Read the model definition and answer for the solid it produces. Units are mm, in the model's axes. A direction names the side the tool comes from. Give positions to 0.01 mm unless a question says otherwise; leave off trailing zeros. Write each loop counter-clockwise with the first axis right and the second up, starting at its lowest first coordinate (ties: lowest second). Pieces come first, ordered by that corner, then holes. Notation, with made-up numbers: (-14.75, -38) -> (-10.75, -38) arc R25 cw to (-10.75, -4) -> close; hole circle Ø8 at (45, -11.75). An arc over 180 degrees is marked (long way). Answer as CSV lines item,"result". Start each with the question number.
1. For a pull along Z with two mould halves and no side action, classify faces 1 (the flat face through (-32.4, 9, -5.3)), 2 (the cylindrical face through (-3.09, 169.89, -4.61)), 3 (the cylindrical face through (-9.634, 5.916, -3.034)) as pulls with the +Z half, pulls with the -Z half, needs draft (parallel to the pull), parting line crosses it, or undercut.
2. The part is cut by section A-A, the plane x = -30.4. Determine the outline of the cut face in (y, z).
3. The part is cut by section D-D, the plane x = 32. Determine the outline of the cut face in (y, z), and give its area (3 significant figures).
4. Find the intervals of material crossed by line 1 (X direction, y = 10.1, z = 0); line 2 (X direction, y = 7, z = 0); line 3 (Z direction, x = -30, y = 10), in increasing order.
5. A tool of negligible diameter and unlimited length cuts with its end or side. For faces 4 (the cylindrical face through (-10.99, 12.27, 0.48)), 5 (the cylindrical face through (-9.634, 100.261, -3.034)), 6 (the flat face through (0, 13, 10.4)), from which of +Z, -Z, +X, -X, +Y, -Y can it reach the whole face along a straight path? Write none if from no direction.
6. Given pin 1 (8 mm diameter, centred on y = 142.5, z = -8, fed in from +X); pin 2 (1.5 mm diameter, centred on x = 8.5, z = -5, fed in from +Y) (3 decimals); pin 3 (3 mm diameter, centred on x = 0, y = 170, fed in from +Z), each flat-ended and moving along its own axis, determine where each tip first touches the part or whether it passes through.
7. The part is cut by section B-B, the plane y = 180. Determine the outline of the cut face in (x, z).
8. The part is cut by section C-C, the plane y = 145. Determine the outline of the cut face in (x, z).
Autodesk Inventor part; units mm, degrees
ref_plane "Płaszczyzna konstrukcyjna1" through (0, 13, 0) normal (0, -1, 0) x (1, 0, 0)
ref_plane "Płaszczyzna konstrukcyjna2" through (0, 12, 0) normal (0, -1, 0) x (1, 0, 0)
ref_plane "YZ Plane" through (0, 0, 0) normal (1, 0, 0) x (0, 1, 0)
sketch "Szkic1" plane through (0, 0, 0) normal (0, 1, 0) x (-1, 0, 0)
  circle A0 centre (0, 0) radius 10.1
  dimension "d0" = 20.2
extrude "Wyciągnięcie proste1" add sketch "Szkic1" along normal blind 200
ref_plane "Płaszczyzna konstrukcyjna1" through (0, 13, 0) normal (0, -1, 0) x (1, 0, 0)
sketch "Szkic2" plane through (0, 13, 0) normal (0, -1, 0) x (1, 0, 0)
  line L0 (0, 0) -> (30.4, 0)
  line L1 (0, 0) -> (30.4, 0) construction
  circle A0 centre (30.4, 0) radius 5.5
  line L2 (35.9, 0) -> (36.9, 0)
  line L3 (36.9, 0) -> (0, 0)
  line L4 (0, 0) -> (0, -6)
  line L5 (0, -6) -> (36.9, -6)
  line L6 (36.9, -6) -> (36.9, 0)
  line L7 (0, 0) -> (0, -16.4984)
  line L8 (0, 6) -> (36.9, 6)
  line L9 (36.9, 6) -> (36.9, 0)
  line L10 (0, 0) -> (-30.4, 0)
  line L11 (0, 0) -> (-30.4, 0) construction
  circle A1 centre (-30.4, 0) radius 5.5
  line L12 (-35.9, 0) -> (-36.9, 0)
  line L13 (-36.9, 0) -> (0, 0)
  line L14 (0, -6) -> (-36.9, -6)
  line L15 (0, 6) -> (-36.9, 6)
  line L16 (-36.9, 6) -> (-36.9, -6)
  line L17 (-24.9, 0) -> (-23.9, 0)
  line L18 (-23.9, 0) -> (-23.9, 6)
  line L19 (-23.9, 0) -> (-23.9, -6)
  line L20 (24.9, 0) -> (23.9, 0)
  line L21 (23.9, 0) -> (23.9, 6)
  line L22 (23.9, 0) -> (23.9, -6)
  dimension "d4" = 30.4
  dimension "d5" = 0
  dimension "d6" = 11
  dimension "d7" = 1
  dimension "d8" = 6
  dimension "d13" = 1
  dimension "d14" = 1
extrude "Wyciągnięcie proste2" add sketch "Szkic2" along normal blind 0.5 contours L10 L18 L15 L8 L21 L0 | L0 L22 L5 L4 | L4 L14 L19 L10 | L21 L8 L9 L2 A0 L0 | L0 A0 L2 L6 L5 L22 | L19 L14 L16 L12 A1 L10 | L10 A1 L12 L16 L15 L18
extrude "Wyciągnięcie proste3" add sketch "Szkic2" against normal blind 4
extrude "Wyciągnięcie proste4" add sketch "Szkic2" along normal blind 4 contours L21 L8 L9 L2 A0 L0 | L0 A0 L2 L6 L5 L22 | L19 L14 L16 L12 A1 L10 | L10 A1 L12 L16 L15 L18
fillet "Zaokrąglenie1" radius 3 8 edges at (-36.9, 13, 6) (-23.9, 10.75, 6) (-36.9, 13, -6) (-23.9, 10.75, -6) (36.9, 13, 6) (23.9, 10.75, 6) (36.9, 13, -6) (23.9, 10.75, -6)
sketch "Szkic3" plane through (0, 0, 0) normal (0, 0, 1) x (1, 0, 0)
  line L0 (10.1, 200) -> (-10.1, 200)
  line L1 (0, 200) -> (0, 190)
  line L2 (0, 190) -> (0, 180)
  line L3 (0, 180) -> (0, 170)
  circle A0 centre (0, 170) radius 2.45
  circle A1 centre (0, 180) radius 2.45
  point P0 (0, 0)
  dimension "d21" = 10
  dimension "d22" = 10
  dimension "d23" = 10
  dimension "d24" = 4.9
  dimension "d25" = 4.9
extrude "Wyciągnięcie proste5" cut sketch "Szkic3" along normal blind 60
pattern_circular "Szyk kołowy1" count 3 over 360 about axis through (0, 0, 0) along (0, 1, 0) of "Wyciągnięcie proste5"
fillet "Zaokrąglenie2" radius 10 1 edges at (10.1, 200, 0)
ref_plane "Płaszczyzna konstrukcyjna2" through (0, 12, 0) normal (0, -1, 0) x (1, 0, 0)
sketch "Szkic4" plane through (0, 12, 0) normal (0, -1, 0) x (1, 0, 0)
  circle A0 centre (0, 0) radius 11
  dimension "d36" = 22
extrude "Wyciągnięcie proste6" add sketch "Szkic4" against normal blind 1
sketch "Szkic5" plane through (0, 0, 0) normal (0, -1, 0) x (1, 0, 0)
  line L0 (0, -2.829) -> (0, 0)
  circle A0 centre (0, 0) radius 2.6
  dimension "d39" = 5.2
extrude "Wyciągnięcie proste7" cut sketch "Szkic5" against normal blind 10
properties part number "andomierz_wal" material "Tworzywo sztuczne ABS"
Results found:
1,face 1,"needs draft"
1,face 2,"undercut"
1,face 3,"parting line crosses it"
2,outline,"(9, -6) -> (17, -6) -> (17, 6) -> (9, 6) -> (9, 5.5) -> (13, 5.5) -> (13, -5.5) -> (9, -5.5) -> close"
3,outline,"(9, -6) -> (17, -6) -> (17, 6) -> (9, 6) -> (9, 5.26) -> (13, 5.26) -> (13, -5.26) -> (9, -5.26) -> close"
3,area,"53.9 mm²"
4,line 1,"x = -36.9 to -35.9, -24.9 to -23.9, -10.1 to 10.1, 23.9 to 24.9, 35.9 to 36.9"
4,line 2,"x = -10.1 to -2.6, 2.6 to 10.1"
4,line 3,"z = -6 to -5.49, 5.49 to 6"
5,face 4,"-Y"
5,face 5,"+Y"
5,face 6,"+Z, +Y"
6,pin 1,"stops at x = 9.27"
6,pin 2,"stops at y = 194.335"
6,pin 3,"stops at z = -2.24"
7,outline,"(-9.71, -2.78) -> (-2.45, 1.41) -> (-2.45, 9.8) arc R10.1 ccw to start; (-7.26, -7.02) arc R10.1 ccw to (7.26, -7.02) -> (0, -2.83) -> close; (2.45, 1.41) -> (9.71, -2.78) arc R10.1 ccw to (2.45, 9.8) -> close"
8,outline,"circle Ø20.2 at (0, 0)"
